```python
from build123d import *

# Parameters (mm, degrees)
BOSS_EXTRUDE1_DEPTH = 3.175
CUT_EXTRUDE1_DEPTH  = 10


with BuildPart() as part:
    # Sketch1 → Boss-Extrude1 (new body)
    with BuildSketch(Plane(origin=(0, 0, 0), x_dir=(1, 0, 0), z_dir=(0, 1, 0))):
        Polygon((0, 0), (53.64, 0), (0, 53.64), align=None)
    extrude(amount=BOSS_EXTRUDE1_DEPTH)

    # Sketch2 → Cut-Extrude1 (cut)
    with BuildSketch(Plane(origin=(0, 3.175, 0), x_dir=(1, 0, 0), z_dir=(0, 1, 0))):
        Polygon((27.04627417, 22.096526702), (29.294873734, 24.345126266), (24.345126266, 29.294873734), (22.096526702, 27.04627417), (23.531953467, 25.610847404), (22.061171363, 24.140065299), (20.802521292, 25.39871537), (18.964043661, 23.560237739), (20.222693732, 22.301587668), (18.758982694, 20.837876631), (20.837876631, 18.758982694), (22.301587668, 20.222693732), (23.560237739, 18.964043661), (25.39871537, 20.802521292), (24.140065299, 22.061171363), (25.610847404, 23.531953467), align=None)
        Polygon((3.175, 30.32), (0, 30.32), (0, 23.32), (3.175, 23.32), (3.175, 25.35), (5.255, 25.35), (5.255, 23.57), (7.855, 23.57), (7.855, 25.35), (9.925, 25.35), (9.925, 28.29), (7.855, 28.29), (7.855, 30.07), (5.255, 30.07), (5.255, 28.29), (3.175, 28.29), align=None)
        Polygon((30.32, 3.175), (30.32, 0), (23.32, 0), (23.32, 3.175), (25.35, 3.175), (25.35, 5.255), (23.57, 5.255), (23.57, 7.855), (25.35, 7.855), (25.35, 9.925), (28.29, 9.925), (28.29, 7.855), (30.07, 7.855), (30.07, 5.255), (28.29, 5.255), (28.29, 3.175), align=None)
    extrude(amount=-CUT_EXTRUDE1_DEPTH, mode=Mode.SUBTRACT)


solid = part.part
```
Could you check a few things on this model? Use its own coordinates, in mm. A direction names the side the tool comes from. Round coordinates to 2 decimals unless told otherwise and drop trailing zeros. Write each loop counter-clockwise with the first axis right and the second up, starting at its lowest first coordinate (ties: lowest second). Pieces come first, ordered by that corner, then holes.
(1) Suppose I cut it at D-D on x = 37. Write out the boundary of the cut face in (y, z) (3 decimals), and give its area (3 significant figures).
Findings below:
outline: (0, -16.64) - (3.175, -16.64) - (3.175, 0) - (0, 0) - close
area: 52.8 mm2
(2) If I drill on probe 1 along Z at (x, y) = (29.5, 1.1) (3 decimals); probe 2 along Z at (x, y) = (3, 0.5); probe 3 along X at (y, z) = (1.3, -5), over which ranges is the centre line in solid material (lowest first)?
Findings below:
probe 1: z = -24.14 to -7.855, -5.255 to -3.175
probe 2: z = -50.64 to -30.32, -23.32 to 0
probe 3: x = 0 to 25.35, 28.29 to 48.64
(3) Suppose I cut it at A-A on x = 4. Write out the boundary of the cut face in (y, z) (3 decimals), and give its area (3 significant figures).
Findings below:
outline: (0, -49.64) - (3.175, -49.64) - (3.175, -28.29) - (0, -28.29) - close; (0, -25.35) - (3.175, -25.35) - (3.175, 0) - (0, 0) - close
area: 148 mm2
(4) Which directions (+Z, -Z, +X, -X, +Y, -Y) give clear straight access to the entire face, cutting with the end or side of a thin tool? Please do faces 4 (the face through (9, 2, -25.35)), 5 (the face through (7, 2, -30.07)), 6 (the face through (41.64, 1.57, -12)), 7 (the face through (28.155, 1.61, -23.205)), 8 (the face through (28.29, 2, -9)).
Findings below:
face 4: -X, +Y, -Y
face 5: +Y, -Y
face 6: -Z, +X, +Y, -Y
face 7: -Z, +Y, -Y
face 8: +Z, +Y, -Y
(5) Suppose I cut it at C-C on z = -35.5. Write out the boundary of the cut face in (x, y) (3 decimals), and give its area (3 significant figures).
Findings below:
outline: (0, 0) - (18.14, 0) - (18.14, 3.175) - (0, 3.175) - close
area: 57.6 mm2
(6) Thinking about a two-plate mould opening in X: for faces 1 (the face through (15, 0, -15)), 2 (the face through (25.35, 2, -4)), 3 (the face through (9.925, 2, -27)), which applies, +X half, -X half, draft (parallel to the pull), parting line (faces both ways), or undercut?
Findings below:
face 1: draft
face 2: undercut
face 3: -X half
(7) For pin 1 (1 mm diameter, centred on x = 27.5, y = 1, fed in from -Z); pin 2 (0.6 mm diameter, centred on y = 1.5, z = -9, fed in from +X); pin 3 (0.5 mm diameter, centred on x = 24, y = 2, fed in from -Z), each with a flat end and sliding along its axis, tell me the tip position at first contact or that it passes through.
Findings below:
pin 1: stops at z = -23.05
pin 2: stops at x = 44.94
pin 3: stops at z = -29.89
(8) Suppose I cut it at B-B on z = -4. Write out the boundary of the cut face in (x, y) (3 decimals).
Findings below:
outline: (0, 0) - (25.35, 0) - (25.35, 3.175) - (0, 3.175) - close; (28.29, 0) - (49.64, 0) - (49.64, 3.175) - (28.29, 3.175) - close
